from build123d import *

# Parameters (mm, degrees)
SKETCH2_W = 3.5
SKETCH2_H = 3.6
FILLET1_R = 0.2
FILLET2_R = 0.6


with BuildPart() as part:
    # Sketch2 → Revolve1 (revolve)
    with BuildSketch(Plane(origin=(0, 0, 0), x_dir=(0, 0, -1), z_dir=(1, 0, 0))):
        with Locations((-4.25, 5.05)):
            Rectangle(SKETCH2_W, SKETCH2_H)
        with BuildLine():
            ThreePointArc((2.5, 6.85), (0, 5.647498436), (-2.5, 6.85))
            Line((-2.5, 6.85), (-2.5, 3.25))
            Line((-2.5, 3.25), (2.5, 3.25))
            Line((2.5, 3.25), (2.5, 6.85))
        make_face()
        with Locations((4.25, 5.05)):
            Rectangle(SKETCH2_W, SKETCH2_H)
    revolve(axis=Axis((0, -6.75, 6), (0, 0, -1)))

    # Fillet1
    fillet1_edges = [part.edges().sort_by_distance(p)[0] for p in [
        (0, -20.35, 6),
        (0, -20.35, -6),
    ]]
    fillet(fillet1_edges, radius=FILLET1_R)

    # Fillet2
    fillet2_edges = [part.edges().sort_by_distance(p)[0] for p in [
        (0, -16.75, -6),
        (0, -16.75, 6),
    ]]
    fillet(fillet2_edges, radius=FILLET2_R)


solid = part.part
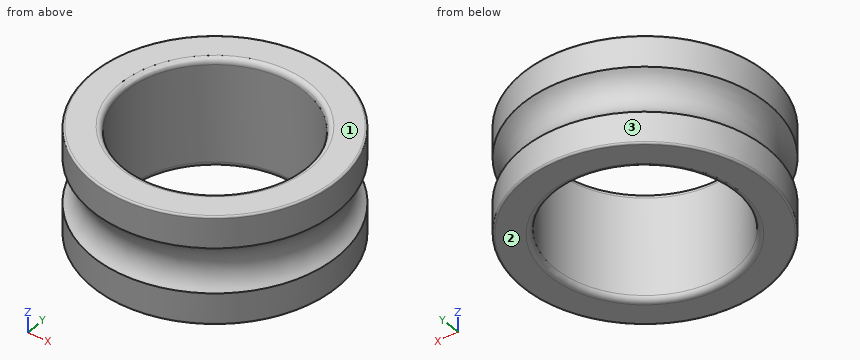
Source: CAD feature listing. Evaluate the final solid. Frame: model axes, mm. Face numbers are marked on the shaded views. Round coordinates to 2 decimals unless told otherwise and drop trailing zeros. Write each loop counter-clockwise with the first axis right and the second up, starting at its lowest first coordinate (ties: lowest second). Pieces come first, ordered by that corner, then holes. Notation, with made-up numbers: M 35,60.25 L 59,60.25 A30 ccw 59,95.25 Z; hole C 78,-35 d8. An arc over 180 degrees is marked long. One line per item, written item: value. Start each with the question number.
Item 1: Section query B-B (y = -6.75). Return the cut outline in (x, z).
Item 2: Mould query, pull axis Z, two halves, no side actions, for the marked faces 1, 2 and 3. Classes: pulls with the +Z half, pulls with the -Z half, needs draft (parallel to the pull), parting line crosses it, or undercut.
Item 3: Section query C-C (z = 5). Return the cut outline in (x, y), plus the area to 3 significant figures.
Item 4: Section query A-A (x = 0). Return the cut outline in (y, z).
Item 5: Ray query, L1, parallel to X at y = -6.75, z = -3; L2, parallel to X at y = -2.5, z = -3.5; L3, parallel to Y at x = 5.5, z = 4.5. Return the intervals inside material, ascending. Write a range as from..to.
Item 6: Section query D-D (z = -0.75). Return the cut outline in (x, y), plus the area to 3 significant figures.
Item 7: Pin query (flat end, axial travel): pin 1 (4 mm diameter, centred on y = 0, z = -0.5, fed in from +X); pin 2 (4 mm diameter, centred on x = 9, z = -5, fed in from +Y). Return the tip coordinate at first contact, or that it passes through.
Result set:
1. outline: M -13.6,-5.8 A0.2 ccw -13.4,-6 L -10.6,-6 A0.6 ccw -10,-5.4 L -10,5.4 A0.6 ccw -10.6,6 L -13.4,6 A0.2 ccw -13.6,5.8 L -13.6,2.5 A3.2 cw -13.6,-2.5 Z; M 10,-5.4 A0.6 ccw 10.6,-6 L 13.4,-6 A0.2 ccw 13.6,-5.8 L 13.6,-2.5 A3.2 cw 13.6,2.5 L 13.6,5.8 A0.2 ccw 13.4,6 L 10.6,6 A0.6 ccw 10,5.4 Z
2. face 1: pulls with the +Z half
2. face 2: pulls with the -Z half
2. face 3: needs draft
3. outline: C 0,-6.75 d27.2; hole C 0,-6.75 d20
3. area: 267 mm²
4. outline: M -20.35,-5.8 A0.2 ccw -20.15,-6 L -17.35,-6 A0.6 ccw -16.75,-5.4 L -16.75,5.4 A0.6 ccw -17.35,6 L -20.15,6 A0.2 ccw -20.35,5.8 L -20.35,2.5 A3.2 cw -20.35,-2.5 Z; M 3.25,-5.4 A0.6 ccw 3.85,-6 L 6.65,-6 A0.2 ccw 6.85,-5.8 L 6.85,-2.5 A3.2 cw 6.85,2.5 L 6.85,5.8 A0.2 ccw 6.65,6 L 3.85,6 A0.6 ccw 3.25,5.4 Z
5. L1: x = -13.6..-10, 10..13.6
5. L2: x = -12.92..-9.05, 9.05..12.92
5. L3: y = -19.19..-15.1, 1.6..5.69
6. outline: C 0,-6.75 d24.97; hole C 0,-6.75 d20
6. area: 176 mm²
7. pin 1: stops at x = 12.02
7. pin 2: stops at y = 4.91
